from build123d import *

# Parameters (mm, degrees)
F0_W     = 11.3
F0_H     = 11.3
F1_DEPTH = 16.4
F2_W     = 11.3
F2_H     = 11.3
F3_DEPTH = 25
F4_R     = 2


with BuildPart() as f1:
    # F0 (on Top) → F1 (new body)
    with BuildSketch(Plane.XY):
        with Locations((5.65, 5.65)):
            Rectangle(F0_W, F0_H)
    extrude(amount=F1_DEPTH)

    # F2 (on face) → F3 (cut)
    with BuildSketch(Plane(origin=(0, 0, 0), x_dir=(0, -1, 0), z_dir=(-1, 0, 0))):
        with Locations((-5.65, 5.65)):
            Rectangle(F2_W, F2_H)
    extrude(amount=-F3_DEPTH, mode=Mode.SUBTRACT)

    # F4
    f4_edges = [f1.edges().sort_by_distance(p)[0] for p in [
        (0, 0, 13.85),
        (11.3, 0, 13.85),
        (0, 11.3, 13.85),
        (11.3, 11.3, 13.85),
    ]]
    fillet(f4_edges, radius=F4_R)


solid = f1.part
CAD build for the part. Positions are in the model's coordinates, mm. Round coordinates to 2 decimals unless told otherwise and drop trailing zeros. Write each loop counter-clockwise with the first axis right and the second up, starting at its lowest first coordinate (ties: lowest second). Pieces come first, ordered by that corner, then holes. Notation, with made-up numbers: M 88.5,43 L 137.5,43 A21 cw 137.5,50 Z; hole C 71,-39 d4. An arc over 180 degrees is marked long. Put each result on its own line as item: value. Start each with the question number.
1) Saw through at C-C, the plane x = 10.25. Write the cut outline in (y, z).
2) Saw through at B-B, the plane x = 1. Write the cut outline in (y, z).
3) Drill centre lines: probe 1 along X at (y, z) = (9.75, 13.7); probe 2 along X at (y, z) = (10.5, 13.1); probe 3 along Y at (x, z) = (0.75, 13.55). Where is each one in solid material? Low to high. Write a range as [from, to].
4) Saw through at A-A, the plane z = 13.85. Write the cut outline in (x, y).
Resolved:
1. outline: M 0.24,11.3 L 11.06,11.3 L 11.06,16.4 L 0.24,16.4 Z
2. outline: M 0.27,11.3 L 11.03,11.3 L 11.03,16.4 L 0.27,16.4 Z
3. probe 1: [0.05, 11.25]
3. probe 2: [0.4, 10.9]
3. probe 3: [0.44, 10.86]
4. outline: M 0,2 A2 ccw 2,0 L 9.3,0 A2 ccw 11.3,2 L 11.3,9.3 A2 ccw 9.3,11.3 L 2,11.3 A2 ccw 0,9.3 Z
